Check sheet for the modelled part. Datum: model origin and axes. Units: mm. A direction names the side the tool comes from. Coordinates: 2 decimals unless noted, no trailing zeros. Write each loop counter-clockwise with the first axis right and the second up, starting at its lowest first coordinate (ties: lowest second). Pieces come first, ordered by that corner, then holes. Notation, with made-up numbers: (-32.75, -34.5) -> (10.25, -34.5) arc R19 cw to (10.25, -21.5) -> close; hole circle Ø10 at (76.25, 56). An arc over 180 degrees is marked (long way). Put each result on its own line as item: value.
```python
from build123d import *

# Parameters (mm, degrees)
SKETCH1_W                              = 400
SKETCH1_H                              = 20
BOSS_EXTRUDE1_DEPTH                    = 12
CBORE_FOR_M8_HEX_HEAD_BOLT1_AT_2_COUNT = 2
CBORE_FOR_M8_HEX_HEAD_BOLT1_AT_2_PITCH = 100
CBORE_FOR_M8_HEX_HEAD_BOLT1_AT_3_COUNT = 2
CBORE_FOR_M8_HEX_HEAD_BOLT1_AT_3_PITCH = 100


with BuildPart() as part:
    # Sketch1 → Boss-Extrude1 (new body)
    with BuildSketch(Plane(origin=(0, 0, 0), x_dir=(1, 0, 0), z_dir=(0, 1, 0))):
        Rectangle(SKETCH1_W, SKETCH1_H)
    extrude(amount=BOSS_EXTRUDE1_DEPTH)

    # Sketch5 → CBORE for M8 Hex Head Bolt1 (revolve, cut)
    with BuildSketch(Plane(origin=(0, 12, 0), x_dir=(0, 0, 1), z_dir=(1, 0, 0))):
        Polygon((0, 0), (0, 12), (4.2, 12), (4.2, 5.3), (9.0055, 5.3), (9.0055, 0.025), (9.0305, 0), align=None)
    cbore_for_m8_hex_head_bolt1 = revolve(axis=Axis((0, 18.35, 0), (0, -1, 0)), mode=Mode.SUBTRACT)

    # CBORE for M8 Hex Head Bolt1 at 2: CBORE for M8 Hex Head Bolt1 ×2
    with Locations(*[(i * CBORE_FOR_M8_HEX_HEAD_BOLT1_AT_2_PITCH, 0, 0) for i in range(1, CBORE_FOR_M8_HEX_HEAD_BOLT1_AT_2_COUNT)]):
        add(cbore_for_m8_hex_head_bolt1, mode=Mode.SUBTRACT)

    # CBORE for M8 Hex Head Bolt1 at 3: CBORE for M8 Hex Head Bolt1 ×2
    with Locations(*[(-i * CBORE_FOR_M8_HEX_HEAD_BOLT1_AT_3_PITCH, 0, 0) for i in range(1, CBORE_FOR_M8_HEX_HEAD_BOLT1_AT_3_COUNT)]):
        add(cbore_for_m8_hex_head_bolt1, mode=Mode.SUBTRACT)


solid = part.part
```
Q1. Material ranges on line 1 along X through (y, z) = (4, -0.75); line 2 along X through (y, z) = (3, 0); line 3 along Z through (x, y) = (0, 10.3), recorded low to high.
Recorded:
line 1: x = -200 to -104.13, -95.87 to -4.13, 4.13 to 95.87, 104.13 to 200
line 2: x = -200 to -104.2, -95.8 to -4.2, 4.2 to 95.8, 104.2 to 200
line 3: z = -10 to -9.01, 9.01 to 10
Q2. Cross-section at A-A (z = 0). State how many separate pieces and enclosed holes the cut face has, plus the area to 3 significant figures.
Recorded:
separate pieces: 4
enclosed holes: 0
area: 4,340 mm2
Q3. Depth check by flat-ended pin: P1, Ø11, axis at x = 0, z = 0, coming from the +Y side. Enter the tip coordinate at first touch or a pass-through.
Recorded:
P1: stops at y = 6.7
Q4. Cross-section at C-C (y = 9.75). Record the cut outline in (x, z), plus the area to 3 significant figures.
Recorded:
outline: (-200, -10) -> (200, -10) -> (200, 10) -> (-200, 10) -> close; hole circle Ø18.01 at (-100, 0); hole circle Ø18.01 at (0, 0); hole circle Ø18.01 at (100, 0)
area: 7,240 mm2
Q5. Tool access check on faces 1 (the flat face through (-3, 0, -5)), 2 (the cylindrical face through (5.48, 9.374, -7.146)). Record the directions out of +Z, -Z, +X, -X, +Y, -Y that give a thin tool (end or side, any length) a straight path to the whole face; none if there is none.
Recorded:
face 1: +Z, -Z, +X, -X, -Y
face 2: +Y
